Here's how the part is built. I have some questions about the finished solid (model axes, mm). Face numbers are marked on the shaded views. A direction names the side the tool comes from. Coordinates: 2 decimals unless noted, no trailing zeros. Order: outer loops, then holes, each group sorted by start corner. A loop starts at its lowest first (then second) coordinate and runs counter-clockwise, first axis right, second up. Notation, with made-up numbers: (35, -6.5) - (60, -6.5) arc R15 cw to (60, 18.5) - close; hole circle Ø7 at (-36, 83). An arc over 180 degrees is marked (long way). Answer in a Markdown table with one row per item. Add a question column.
Item 1: Thinking about a two-plate mould opening in X: for the marked faces 5, 6 and 7, which applies, +X half, -X half, draft (parallel to the pull), parting line (faces both ways), or undercut?
Item 2: I want a section at B-B (z = 47). Please give me the cut outline in (x, y), plus the area to 3 significant figures.
Item 3: Will these pins go through, and if not, where does the flat tip stop? pin 1 Ø6 at (x, z) = (-27.5, 34.5) entering from -Y; pin 2 Ø4 at (x, y) = (-17, -7) entering from +Z; pin 3 Ø8 at (y, z) = (-36.5, 30.5) entering from -X.
Item 4: On a 3-axis mill with a long thin cutter (end or side, diameter ignored), from which of +Z, -Z, +X, -X, +Y, -Y can I reach the whole of each face in a straight line? I mean the marked faces 1, 2, 3 and 4. Say none if no direction works.
Item 5: I want a section at A-A (z = 39). Please give me the cut outline in (x, y), plus the area to 3 significant figures.
```python
from build123d import *

# Parameters (mm, degrees)
F1_DEPTH = 25
F3_R     = 7.7623093382
F4_DEPTH = 25


with BuildPart() as f1:
    # F0 (on Front) → F1 (new body)
    with BuildSketch(Plane.XZ):
        Polygon((25.9043528415, 51.4944938206), (23.085501045, 53.0769191682), (-10.6548462063, -5.9193591587), (-27.623673901, -5.9193591587), (-27.623673901, -22.8881891817), (-10.6548462063, -22.8881891817), (-10.6548462063, -12.4306539074), align=None)
    extrude(amount=F1_DEPTH)

    # F1_face (on face) → F2 (revolve)
    with BuildSketch(Plane(origin=(-7.5947034843, -25, 1.5087803319), x_dir=(1, 0, 0), z_dir=(0, -1, 0))):
        Polygon((33.4990563258, 49.9857134887), (30.6802045293, 51.5681388363), (-3.060142722, -7.4281394906), (-20.0289704167, -7.4281394906), (-20.0289704167, -24.3969695136), (-3.060142722, -24.3969695136), (-3.060142722, -13.9394342393), align=None)
    revolve(axis=Axis((-27.623673901, -25, -14.4037741702), (0, 0, -1)))

    # F3 (on face) → F4 (cut)
    with BuildSketch(Plane(origin=(0, 0, -22.8881891817), x_dir=(1, 0, 0), z_dir=(0, 0, -1))):
        with Locations((-26.4316089451, 28.0019678175)):
            Circle(F3_R)
    extrude(amount=-F4_DEPTH, mode=Mode.SUBTRACT)


solid = f1.part
```
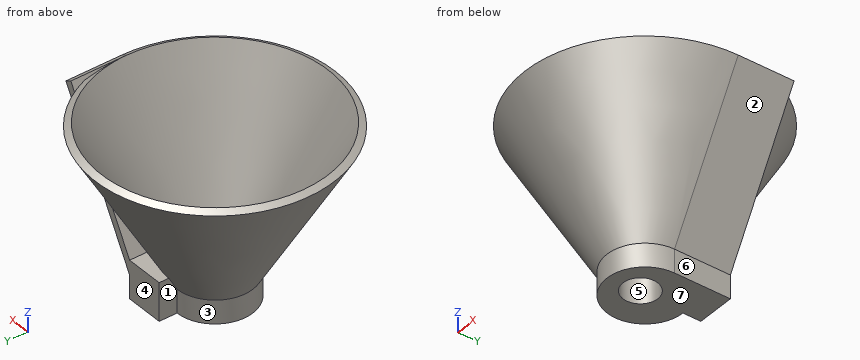
Values follow:
| question | item | result |
|---|---|---|
| 1 | face 5 | undercut |
| 1 | face 6 | +X half |
| 1 | face 7 | draft |
| 2 | outline | (19.61, -5.88) arc R50.96 ccw (long way) to (23.33, -25) - (23.33, 0) - (19.61, 0) - close; hole circle Ø94.47 at (-27.62, -25) |
| 2 | area | 1,190 mm^2 |
| 3 | pin 1 | stops at y = -70.52 |
| 3 | pin 2 | stops at z = 4.45 |
| 3 | pin 3 | stops at x = -70.1 |
| 4 | face 1 | -Z, -X, +Y |
| 4 | face 2 | -Z, +X, +Y, -Y |
| 4 | face 3 | -Z |
| 4 | face 4 | -Z, +X, +Y |
| 5 | outline | (15.03, -6.79) arc R46.38 ccw (long way) to (18.76, -25) - (18.76, 0) - (15.03, 0) - close; hole circle Ø85.32 at (-27.62, -25) |
| 5 | area | 1,090 mm^2 |
